Autodesk Fusion 360 part; units mm, degrees
sketch "Boceto1" plane through (0, 0, 0) normal (0, 0, 1) x (1, 0, 0)
  line L0 (-25.6714, 0) -> (25.6714, 0) construction
  line L1 (0, -23) -> (0, 29) construction
  line L2 (-3.5, 21.001) -> (3.5, 21.001) construction
  line L3 (-4, 25.5) -> (4, 25.5) construction
  arc A0 (3.5, 25.5) -> (-3.5, 25.5) centre (0, 25.5) ccw
  line L4 (-3.5, 25.5) -> (-3.5, -29.5)
  line L5 (3.5, 25.5) -> (3.5, -29.5)
  line L6 (-4, -29.5) -> (4, -29.5) construction
  arc A1 (-3.5, -29.5) -> (3.5, -29.5) centre (0, -29.5) ccw
  circle A2 centre (0, -29.5) radius 2
  circle A3 centre (0, -16.762) radius 2
  line L7 (-1.9722, 25.5) -> (-1.9722, 10.5)
  line L8 (2.0278, 25.5) -> (2.0278, 10.5)
  arc A4 (2.0278, 25.5) -> (-1.9722, 25.5) centre (0.0278, 25.5) ccw
  arc A5 (-1.9722, 10.5) -> (2.0278, 10.5) centre (0.0278, 10.5) ccw
  point P0 (-3.5, 0)
  point P1 (3.5, -0.1376)
  point P2 (0, 21.001)
  point P3 (0, 21.001)
  point P4 (0, -33)
  dimension "d4" = 7
  dimension "d6" = 4
  dimension "d7" = 4
  dimension "d8" = 12.738
  dimension "d9" = 15
  dimension "d10" = 15
  dimension "d11" = 4
  dimension "d14" = 55
  dimension "d15" = 62
extrude "Extruir1" add sketch "Boceto1" along normal blind 3
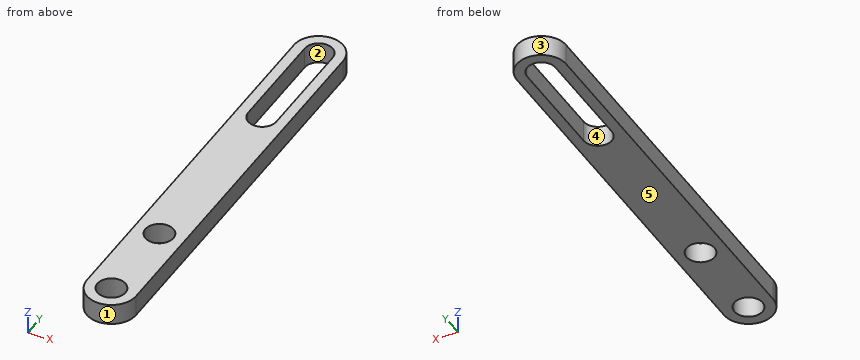
Part model, mm, in its own coordinate system. Face numbers are marked on the shaded views. A direction names the side the tool comes from. Give positions to 0.01 mm unless a question says otherwise; leave off trailing zeros. Loops run counter-clockwise (first coordinate to the right, second up) from the corner with the lowest first, then second, coordinate; pieces in that order, holes last. Notation, with made-up numbers: M 56,55 L 89,55 A11 cw 89,64 Z; hole C 20.25,-17 d11. An arc over 180 degrees is marked long. Put each result on its own line as item: value. Start each with the question number.
1) Probe probe 1 along Y at (x, z) = (0, 1.05); probe 2 along X at (y, z) = (16.5, 2.35); probe 3 along Y at (x, z) = (-1, 1.55). List the from-to ranges inside material, lowest first.
2) Saw through at B-B (x = 0). List the corners of the cut face in (y, z).
3) Pull direction X, two halves, no side cores. Call the marked faces 3, 4 and 5: +X half, -X half, draft (parallel to the pull), parting line (faces both ways), or undercut.
4) Saw through at D-D (x = -2.75). List the corners of the cut face in (y, z), then the cut area to 3 significant figures.
5) Saw through at A-A (y = 23). List the corners of the cut face in (x, z), then the cut area to 3 significant figures.
6) 3-axis set-ups, long thin cutter, end or side, ignore diameter. For the marked faces 1 and 2: which of +Z, -Z, +X, -X, +Y, -Y reach the whole face in a straight line?
7) Saw through at C-C (z = 2.25). List the corners of the cut face in (x, y).
Numbers:
1. probe 1: -33 to -31.5, -27.5 to -18.76, -14.76 to 8.5, 27.5 to 29
1. probe 2: -3.5 to -1.97, 2.03 to 3.5
1. probe 3: -32.85 to -31.23, -27.77 to -18.49, -15.03 to 8.78, 27.22 to 28.85
2. outline: M -33,0 L -31.5,0 L -31.5,3 L -33,3 Z; M -27.5,0 L -18.76,0 L -18.76,3 L -27.5,3 Z; M -14.76,0 L 8.5,0 L 8.5,3 L -14.76,3 Z; M 27.5,0 L 29,0 L 29,3 L 27.5,3 Z
3. face 3: parting line
3. face 4: undercut
3. face 5: draft
4. outline: M -31.67,0 L 27.67,0 L 27.67,3 L -31.67,3 Z
4. area: 178 mm^2
5. outline: M -3.5,0 L -1.97,0 L -1.97,3 L -3.5,3 Z; M 2.03,0 L 3.5,0 L 3.5,3 L 2.03,3 Z
5. area: 9.00 mm^2
6. face 1: +Z, -Z, -Y
6. face 2: +Z, -Z
7. outline: M -3.5,-29.5 A3.5 ccw 3.5,-29.5 L 3.5,25.5 A3.5 ccw -3.5,25.5 Z; hole C 0,-29.5 d4; hole C 0,-16.76 d4; hole M -1.97,10.5 A2 ccw 2.03,10.5 L 2.03,25.5 A2 ccw -1.97,25.5 Z
